Source: three-view drawing plus pictorial views. Frame: mm from the lowest corner of the part. A direction names the side the tool comes from. Give positions to 0.01 mm unless a question says otherwise; leave off trailing zeros. Order: outer loops, then holes, each group sorted by start corner. A loop starts at its lowest first (then second) coordinate and runs counter-clockwise, first axis right, second up. Notation, with made-up numbers: (84, 11.5) -> (100, 11.5) arc R22 cw to (100, 36.5) -> close; hole circle Ø8 at (45, 81). An arc over 180 degrees is marked (long way). Write item = value, one per line.
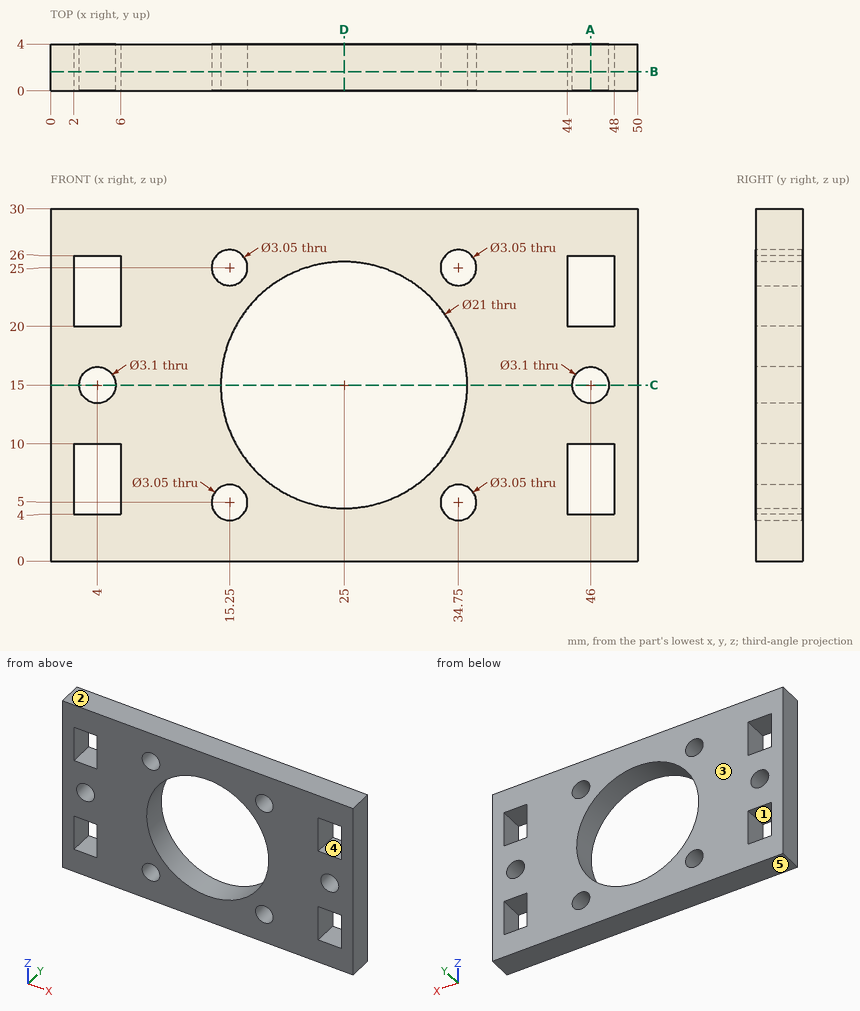
1) Section query C-C (z = 15). Output: boundary loops of the cut face in (x, y).
Check sheet entries:
outline = (0, 0) -> (2.45, 0) -> (2.45, 4) -> (0, 4) -> close; (5.55, 0) -> (14.5, 0) -> (14.5, 4) -> (5.55, 4) -> close; (35.5, 0) -> (44.45, 0) -> (44.45, 4) -> (35.5, 4) -> close; (47.55, 0) -> (50, 0) -> (50, 4) -> (47.55, 4) -> close
2) First-contact query: P1, Ø1.5, axis at y = 1, z = 16.5, coming from the -X side. Flat tip, straight axial feed; report the tip coordinate or a pass-through.
Check sheet entries:
P1 = 0
3) Mould query, pull axis Z, two halves, no side actions, for the marked faces 3, 4 and 5. Classes: +Z half, -Z half, draft (parallel to the pull), parting line (faces both ways), or undercut.
Check sheet entries:
face_3 = draft
face_4 = undercut
face_5 = -Z half
4) Section query B-B (y = 1.65). Count the separate pieces of the cut face and the enclosed holes in it, plus the area to 3 significant figures.
Check sheet entries:
separate_pieces = 1
enclosed_holes = 11
area = 1,010 mm²
5) Reachability of the marked faces 1 and 2 from +Z, -Z, +X, -X, +Y, -Y: full face, straight path, thin tool, end or side. Return the list, or none.
Check sheet entries:
face_1 = +Y, -Y
face_2 = +Z, +X, -X, +Y, -Y
6) Section query A-A (x = 46). Output: boundary loops of the cut face in (y, z).
Check sheet entries:
outline = (0, 0) -> (4, 0) -> (4, 4) -> (0, 4) -> close; (0, 10) -> (4, 10) -> (4, 13.45) -> (0, 13.45) -> close; (0, 16.55) -> (4, 16.55) -> (4, 20) -> (0, 20) -> close; (0, 26) -> (4, 26) -> (4, 30) -> (0, 30) -> close
7) Line query: line 1 (X direction, y = 2.1, z = 26.25); line 2 (Z direction, x = 46, y = 2.5); line 3 (X direction, y = 3.1, z = 8). Output: solid intervals per line, ascending. Write a range as from..to.
Check sheet entries:
line_1 = 0..14.38, 16.12..33.88, 35.62..50
line_2 = 0..4, 10..13.45, 16.55..20, 26..30
line_3 = 0..2, 6..17.17, 32.83..44, 48..50
8) Section query D-D (x = 25). Output: boundary loops of the cut face in (y, z).
Check sheet entries:
outline = (0, 0) -> (4, 0) -> (4, 4.5) -> (0, 4.5) -> close; (0, 25.5) -> (4, 25.5) -> (4, 30) -> (0, 30) -> close
